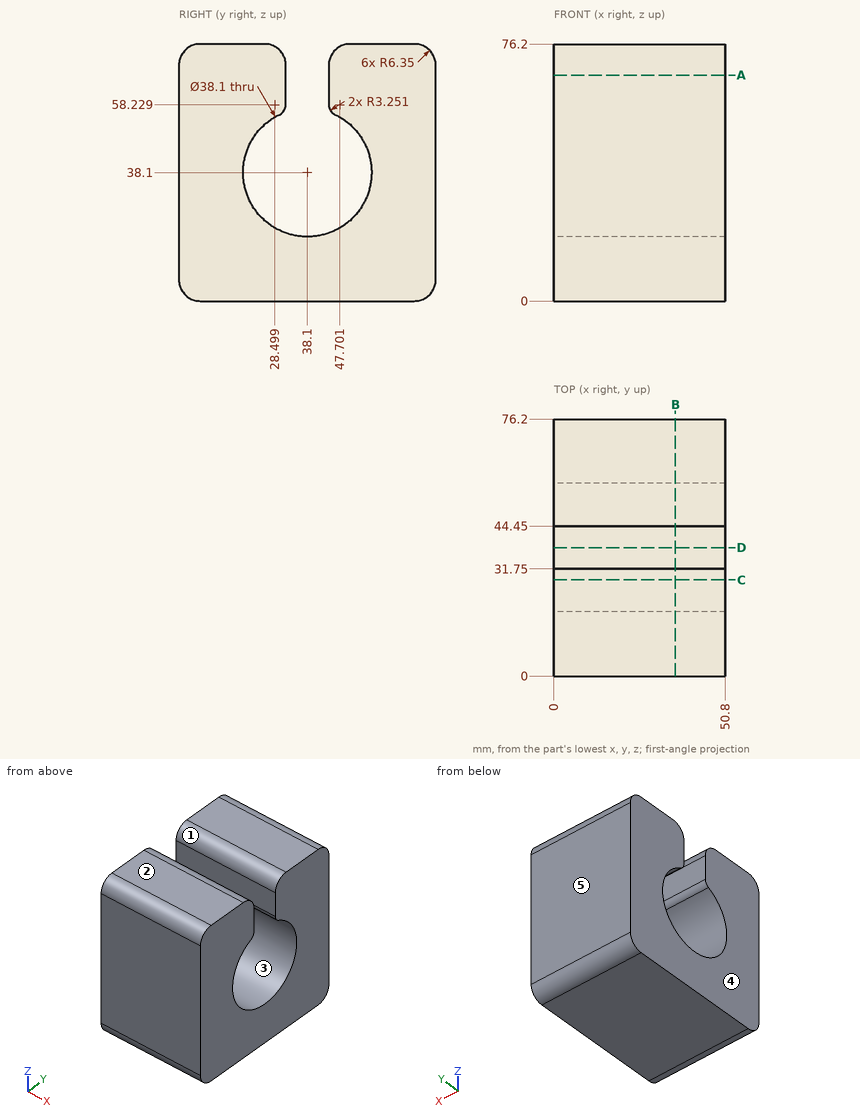
Job drawing, mm, ordinate dimensions from the low corner. One solid piece. A direction names the side the tool comes from. Give positions to 0.01 mm unless a question says otherwise; leave off trailing zeros. Write each loop counter-clockwise with the first axis right and the second up, starting at its lowest first coordinate (ties: lowest second). Pieces come first, ordered by that corner, then holes. Notation, with made-up numbers: M -3.5,34 L 48.5,34 A21 cw 48.5,68 Z; hole C 75,-39.5 d11. An arc over 180 degrees is marked long. Put each result on its own line as item: value. Start each with the question number.
(1) Mould opens along Y. For the marked faces 3, 4 and 5 say: +Y half, -Y half, draft (parallel to the pull), parting line (faces both ways), or undercut.
(2) Band-saw the part on B-B, the plane x = 36. Write the cut outline in (y, z).
(3) Flat gauge pins, fed straight in: pin 1 Ø6 at (y, z) = (20.5, 65) entering from -X; pin 2 Ø12 at (y, z) = (38, 46.5) entering from +X. Where does each tip first touch, or does it go through?
(4) Band-saw the part on A-A, the plane z = 67. Write the cut outline in (x, y).
(5) Band-saw the part on D-D, the plane y = 38.1. Write the cut outline in (x, z).
(6) Which spindle directions (+Z, -Z, +X, -X, +Y, -Y) get a long thin tool onto all of the face, cutting with end or side? Do the marked faces 1 and 2. Say none if no direction does.
(7) Band-saw the part on C-C, the plane y = 28.5. Write the cut outline in (x, z) (1 decimal), and give its area (3 significant figures).
(8) Probe L1, parallel to Y at x = 28, z = 38.1; L2, parallel to Y at x = 11, z = 66; L3, parallel to Z at x = 18, y = 70. List the from-to ranges inside material, lowest first.
Response values:
1. face 3: undercut
1. face 4: draft
1. face 5: +Y half
2. outline: M 0,6.35 A6.35 ccw 6.35,0 L 69.85,0 A6.35 ccw 76.2,6.35 L 76.2,69.85 A6.35 ccw 69.85,76.2 L 50.8,76.2 A6.35 ccw 44.45,69.85 L 44.45,58.23 A3.25 ccw 46.3,55.29 A19.05 cw long 29.9,55.29 A3.25 ccw 31.75,58.23 L 31.75,69.85 A6.35 ccw 25.4,76.2 L 6.35,76.2 A6.35 ccw 0,69.85 Z
3. pin 1: stops at x = 0
3. pin 2: passes through
4. outline: M 0,0 L 50.8,0 L 50.8,31.75 L 0,31.75 Z; M 0,44.45 L 50.8,44.45 L 50.8,76.2 L 0,76.2 Z
5. outline: M 0,0 L 50.8,0 L 50.8,19.05 L 0,19.05 Z
6. face 1: +Z, +X, -X
6. face 2: +Z, +X, -X, +Y, -Y
7. outline: M 0,0 L 50.8,0 L 50.8,21.6 L 0,21.6 Z; M 0,54.6 L 50.8,54.6 L 50.8,75.4 L 0,75.4 Z
7. area: 2,160 mm2
8. L1: y = 0 to 19.05, 57.15 to 76.2
8. L2: y = 0 to 31.75, 44.45 to 76.2
8. L3: z = 0 to 76.2
